Autodesk Inventor part; units mm, degrees
ref_plane "YZ Plane" through (0, 0, 0) normal (1, 0, 0) x (0, 1, 0)
ref_plane "XZ Plane" through (0, 0, 0) normal (0, 1, 0) x (-1, 0, 0)
ref_plane "XY Plane" through (0, 0, 0) normal (0, 0, 1) x (1, 0, 0)
sketch "Sketch1" plane through (0, 0, 0) normal (0, 0, 1) x (1, 0, 0)
  circle A0 centre (0, 0) radius 15.875
  line L0 (0, 0) -> (-127, 0)
  circle A1 centre (-127, 0) radius 15.875
  line L1 (-127, 15.875) -> (0, 15.875)
  line L2 (0, -15.875) -> (-127, -15.875)
  circle A2 centre (-127, 0) radius 2.1082
  dimension "d0" = 31.75
  dimension "d1" = 127
  dimension "d2" = 31.75
  dimension "d3" = 4.2164
extrude "Extrusion1" add sketch "Sketch1" along normal blind 3.175
sketch "Sketch2" plane through (0, 0, 0) normal (0, 0, -1) x (-1, 0, 0)
  arc A0 (127, -15.875) -> (127, 15.875) centre (127, 0) ccw
  line L0 (0, 15.875) -> (127, 15.875)
  arc A1 (0, 15.875) -> (0, -15.875) centre (0, 0) ccw
  line L1 (127, -15.875) -> (0, -15.875)
  circle A2 centre (127, 0) radius 2.1082
  line L2 (130.175, -3.175) -> (123.825, -3.175)
  line L3 (123.825, -3.175) -> (123.825, 3.175)
  line L4 (123.825, 3.175) -> (130.175, 3.175)
  line L5 (130.175, 3.175) -> (130.175, -3.175)
  line L6 (130.175, -3.175) -> (123.825, 3.175) construction
  line L7 (123.825, -3.175) -> (130.175, 3.175) construction
  dimension "d25" = 6.35
  dimension "d26" = 6.35
extrude "Extrusion2" add sketch "Sketch2" along normal blind 6.35 contours L1 A1 L0 A0
fillet "Fillet1" radius 3.175 4 edges at (15.875, 0, -6.35) (-63.5, -15.875, -6.35) (-142.875, 0, -6.35) (-63.5, 15.875, -6.35)
sketch "Sketch3" plane through (0, 0, 3.175) normal (0, 0, 1) x (1, 0, 0)
  arc A0 (-127, 15.875) -> (-127, -15.875) centre (-127, 0) ccw
  line L0 (-127, -15.875) -> (0, -15.875)
  arc A1 (0, -15.875) -> (0, 15.875) centre (0, 0) ccw
  line L1 (0, 15.875) -> (-127, 15.875)
  circle A2 centre (-127, 0) radius 2.1082
  circle A3 centre (-127, 0) radius 3.9688
  dimension "d10" = 7.9375
extrude "Extrusion3" add sketch "Sketch3" along normal blind 3.175 contours L1 A1 L0 A0
sketch "Sketch4" plane through (0, 0, 6.35) normal (0, 0, 1) x (1, 0, 0)
  line L0 (-127, -15.875) -> (0, -15.875)
  arc A0 (0, -15.875) -> (0, 15.875) centre (0, 0) ccw
  line L1 (0, 15.875) -> (-127, 15.875)
  arc A1 (-127, 15.875) -> (-127, -15.875) centre (-127, 0) ccw
  circle A2 centre (-127, 0) radius 3.9688
  circle A3 centre (-127, 0) radius 2.1082
  circle A4 centre (-127, 0) radius 11.1125
  circle A5 centre (0, 0) radius 11.1125
  dimension "d13" = 22.225
  dimension "d14" = 22.225
extrude "Extrusion4" add sketch "Sketch4" along normal blind 5.5372 contours A1 L1 A0 L0
sketch "Sketch5" plane through (0, 0, 11.8872) normal (0, 0, 1) x (1, 0, 0)
  circle A0 centre (-76.2, 0) radius 2.1082
  circle A1 centre (-50.8, 0) radius 2.1082
  circle A2 centre (-127, 0) radius 2.1082
  point P0 (0, 0)
  dimension "d17" = 4.2164
  dimension "d18" = 4.2164
  dimension "d19" = 50.8
  dimension "d20" = 50.8
extrude "Extrusion5" cut sketch "Sketch5" against normal blind 25.4 contours A0 | A1
fillet "Fillet2" radius 1.5875 4 edges at (-142.875, 0, 11.8872) (-63.5, -15.875, 11.8872) (15.875, 0, 11.8872) (-63.5, 15.875, 11.8872)
fillet "Fillet3" radius 1.5875 1 edges at (-130.9688, 0, 6.35)
properties part number "Plate E"
Here's how the part is built. I have some questions about the finished solid (model axes, mm). A direction names the side the tool comes from. Coordinates: 2 decimals unless noted, no trailing zeros. Use CSV: the item, a comma, the result in double quotes. Start each with the question number.
1. For faces 1 (the face through (-125, -2, 3.175)), 2 (the face through (-65, 0, 11.887)), 3 (the face through (-127, -3.175, -3)), which set-ups out of +Z, -Z, +X, -X, +Y, -Y let a thin tool reach every point of the face, with its end or its side?
2. Suppose I cut it at B-B on z = 8.75. Give the number of separate pieces and of enclosed holes in the cut face, then the cut area to 3 significant figures.
3. If we mould it in two halves opening along Y, with no side actions, what happens to faces 4 (the face through (-142.87, -0.35, 3.47)), 5 (the face through (-64, -15.875, 3)), 6 (the face through (-52.473, -1.283, 2.896))? For each: +Y half, -Y half, draft (parallel to the pull), parting line (faces both ways), or undercut.
4. Please list where these lines run through material, in increasing order: line 1 (X direction, y = -6, z = 7.5); line 2 (X direction, y = -1, z = 2.75); line 3 (Y direction, x = 0, z = 8.5) (1 decimal). Write a range as from..to.
5. I'm going to push flat-ended pins straight in: pin 1 (11 mm diameter, centred on x = -122, y = -0.5, fed in from +Z); pin 2 (7 mm diameter, centred on x = -127, y = 0, fed in from +Z) (3 decimals); pin 3 (6 mm diameter, centred on y = 4, z = -1.5, fed in from +X). Where does each tip first touch, or does it pass through?
Output:
1,face 1,"+Z"
1,face 2,"+Z, +X, -X, +Y, -Y"
1,face 3,"-Z"
2,separate pieces,"1"
2,enclosed holes,"4"
2,area,"4,020 mm2"
3,face 4,"parting line"
3,face 5,"-Y half"
3,face 6,"undercut"
4,line 1,"x = -141.7..-136.35, -117.65..-9.35, 9.35..14.7"
4,line 2,"x = -142.84..-128.86, -125.14..-78.06, -74.34..-52.66, -48.94..15.84"
4,line 3,"y = -15.9..-11.1, 11.1..15.9"
5,pin 1,"stops at z = 6.35"
5,pin 2,"stops at z = 3.175"
5,pin 3,"stops at x = 15.84"
